Can you work these out from the model? Positions are in its coordinate system, mm. A direction names the side the tool comes from. Coordinates: 2 decimals unless noted, no trailing zeros. Loops run counter-clockwise (first coordinate to the right, second up) from the corner with the lowest first, then second, coordinate; pieces in that order, holes last. Notation, with made-up numbers: M 87,-38.5 L 143,-38.5 A26 cw 143,-7.5 Z; hole C 67,-18.75 d4. An arc over 180 degrees is marked long. Return JSON: item names as keys, results as strings. Group by question number.
```python
from build123d import *

# Parameters (mm, degrees)
BOSS_EXTRUDE1_DEPTH      = 20
BOSS_EXTRUDE1_DEPTH_BACK = 5
BOSS_EXTRUDE2_START      = -5
BOSS_EXTRUDE2_DEPTH      = 5
BOSS_EXTRUDE3_REACH      = 316.977


with BuildPart() as part:
    # Sketch1 → Boss-Extrude1 (new, two sides: drawn at the far end of the back side and taken through both)
    with BuildSketch(Plane(origin=(0, 0, 0), x_dir=(1, 0, 0), z_dir=(0, 1, 0)).offset(-BOSS_EXTRUDE1_DEPTH_BACK)):
        with BuildLine():
            Line((0, 25), (0, 22.5))
            ThreePointArc((0, 22.5), (-22.5, 0), (0, -22.5))
            Line((0, -22.5), (0, -25))
            ThreePointArc((0, -25), (-25, 0), (0, 25))
        make_face()
    extrude(amount=BOSS_EXTRUDE1_DEPTH + BOSS_EXTRUDE1_DEPTH_BACK)

    # Sketch2 → Boss-Extrude2 (add)
    with BuildSketch(Plane(origin=(0, 0, 0), x_dir=(1, 0, 0), z_dir=(0, 1, 0)).offset(BOSS_EXTRUDE2_START)):
        with BuildLine():
            Line((0, -25), (0, -180))
            ThreePointArc((0, -180), (-172.249721603, -52.249721603), (-100, 149.666295471))
            Line((-100, 149.666295471), (-100, 185.5))
            Line((-100, 185.5), (0, 185.5))
            Line((0, 185.5), (0, 25))
            ThreePointArc((0, 25), (-25, 0), (0, -25))
        make_face()
    extrude(amount=BOSS_EXTRUDE2_DEPTH)


with BuildPart() as body_2:
    # Mirror1: mirrored copy
    add(part.part.mirror(Plane.ZX.offset(-82.5)))

    # Sketch3 → Boss-Extrude3 (add, up to next)
    with BuildSketch(Plane.XZ.offset(5), mode=Mode.PRIVATE) as boss_extrude3_sk1:
        with BuildLine():
            Line((-100, -149.666295471), (-100, -185.5))
            Line((-100, -185.5), (-80, -185.5))
            Line((-80, -185.5), (-80, -149.666295471))
            ThreePointArc((-80, -149.666295471), (-164.619580528, 41.235830377), (0, 169.705627485))
            Line((0, 169.705627485), (0, 180))
            ThreePointArc((0, 180), (-172.249721603, 52.249721603), (-100, -149.666295471))
        make_face()
    boss_extrude3_tool1 = extrude(boss_extrude3_sk1.sketch, amount=BOSS_EXTRUDE3_REACH, mode=Mode.PRIVATE) - body_2.part

    add(part.part)  # Boss-Extrude3 merges part
    add(boss_extrude3_tool1.solids().sort_by_distance((-95.92581, -5, -167.583148))[0])


solid = body_2.part
```
1) Suppose I cut it at C-C, the plane y = -49. List the corners of the cut face in (x, z) for me, then the cut area to 3 significant figures.
2) If we mould it in two halves opening along Y, with no side actions, what happens to faces 1 (the face through (-69, -165, -5)), 2 (the face through (-165.356, -81.415, 38.174)), 3 (the face through (0, -82, 177))? For each: +Y half, -Y half, draft (parallel to the pull), parting line (faces both ways), or undercut.
3) If I drill on line 1 (Y direction, x = -57, z = 147); line 2 (Y direction, x = -82, z = -149.5); line 3 (X direction, y = -99, z = -54.5), over which ranges is the centre line in solid material (lowest first)? Write a range as from..to.
4) Suppose I cut it at D-D, the plane x = -13.5. List the corners of the cut face in (y, z) for me.
5) For faces 4 (the face through (-24.994, -174.86, 0.55)), 5 (the face through (-100, -81, -167)), 6 (the face through (-65, -5, -10)), 7 (the face through (-24.994, 9.86, 0.55)), which set-ups out of +Z, -Z, +X, -X, +Y, -Y let a thin tool reach every point of the face, with its end or its side?
6) Suppose I cut it at B-B, the plane x = -134.5. List the corners of the cut face in (y, z) for me.
7) Suppose I cut it at A-A, the plane z = 0. List the corners of the cut face in (x, y) for me, then the cut area to 3 significant figures.
8) For pin 1 (5 mm diameter, centred on y = -44.5, z = -62, fed in from +X); pin 2 (5 mm diameter, centred on x = -112.5, z = -119, fed in from -Y); pin 3 (1.5 mm diameter, centred on y = -46.5, z = 101.5, fed in from -X), each with a flat end and sliding along its axis, tell me the tip position at first contact or that it passes through.
Returned:
{
 "1": {"outline": "M -100,-185.5 L -80,-185.5 L -80,-149.67 A169.71 cw 0,169.71 L 0,180 A180 ccw -100,-149.67 Z", "area": "5,390 mm²"},
 "2": {"face 1": "-Y half", "face 2": "undercut", "face 3": "draft"},
 "3": {"line 1": "y = -165..-160, -5..0", "line 2": "y = -165..0", "line 3": "x = -171.55..-160.72"},
 "4": {"outline": "M -185,-21.04 L -165,-21.04 L -165,-185.5 L -160,-185.5 L -160,-18 L -185,-18 Z; M -185,18 L -160,18 L -160,169.17 L -5,169.17 L -5,18 L 20,18 L 20,21.04 L 0,21.04 L 0,179.49 L -165,179.49 L -165,21.04 L -185,21.04 Z; M -5,-185.5 L 0,-185.5 L 0,-21.04 L 20,-21.04 L 20,-18 L -5,-18 Z"},
 "5": {"face 4": "-X, -Y", "face 5": "-Z, -X, +Y, -Y", "face 6": "+X", "face 7": "-X, +Y"},
 "6": {"outline": "M -165,-119.62 L 0,-119.62 L 0,119.62 L -165,119.62 Z; hole M -160,-103.49 L -5,-103.49 L -5,103.49 L -160,103.49 Z"},
 "7": {"outline": "M -180,-165 L -25,-165 L -25,-185 L -22.5,-185 L -22.5,-160 L -169.71,-160 L -169.71,-5 L -22.5,-5 L -22.5,20 L -25,20 L -25,0 L -180,0 Z", "area": "3,270 mm²"},
 "8": {"pin 1": "stops at x = -156.97", "pin 2": "stops at y = -165", "pin 3": "stops at x = -149.16"}
}
